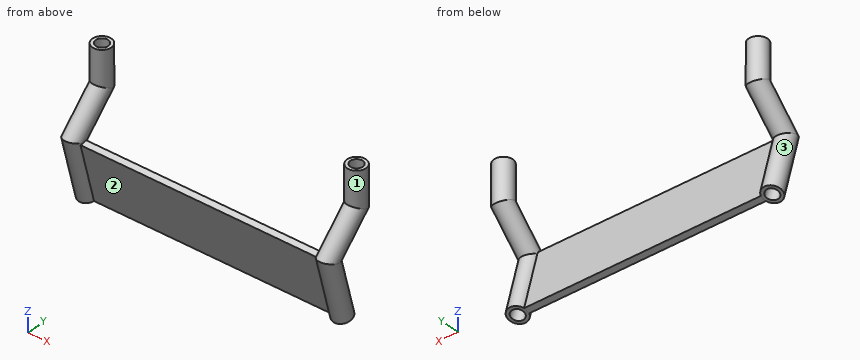
```python
from build123d import *

# Parameters (mm, degrees)
SWEEP_THIN1_PROFILE_R   = 30
SWEEP_THIN1_PROFILE_R_2 = 20
EXTRUDE_THIN1_START     = 20
EXTRUDE_THIN1_DEPTH     = 760


with BuildPart() as part:
    # Sweep-Thin1: sweep along a path in Sketch21
    with BuildLine(Plane(origin=(0, 0, 0), x_dir=(0, 0, -1), z_dir=(1, 0, 0))) as sweep_thin1_path:
        Line((0, 0), (120, 0))
        Line((120, 0), (226.066017178, -106.066017178))
        Line((226.066017178, -106.066017178), (419.251182436, -54.302208157))
    # Sweep-Thin1 profile (on start of the path) → Sweep-Thin1 (sweep)
    with BuildSketch(Plane(origin=(0, 0, 0), x_dir=(-1, 0, 0), z_dir=(0, 0, -1))):
        Circle(SWEEP_THIN1_PROFILE_R)
        Circle(SWEEP_THIN1_PROFILE_R_2, mode=Mode.SUBTRACT)
    sweep_thin1 = sweep(path=sweep_thin1_path.line, transition=Transition.RIGHT)

    # Sketch32 → Extrude-Thin1 (add)
    with BuildSketch(Plane(origin=(0, 0, 0), x_dir=(0, 0, -1), z_dir=(1, 0, 0)).offset(EXTRUDE_THIN1_START)):
        Polygon((228.654207629, -115.725275441), (421.839372887, -63.96146642), (416.662991985, -44.642949895), (223.477826727, -96.406758915), align=None)
    extrude(amount=EXTRUDE_THIN1_DEPTH)

    # Mirror1: Sweep-Thin1 across plane
    add(sweep_thin1.mirror(Plane(origin=(404.142135624, 0, 0), x_dir=(0, 0, 1), z_dir=(1, 0, 0))))


solid = part.part
```
Verification items for the finished model (mm, model axes). Face numbers are marked on the shaded views. A direction names the side the tool comes from. Give positions to 0.01 mm unless a question says otherwise; leave off trailing zeros. Loops run counter-clockwise (first coordinate to the right, second up) from the corner with the lowest first, then second, coordinate; pieces in that order, holes last.
1. Thickness scan on line 1 (Y direction, x = 0, z = -95); line 2 (X direction, y = 18.5, z = -112.5); line 3 (X direction, y = -60, z = -185.5). Record the ranges inside material, lowest first.
2. Section check A-A, the plane x = 0. Enter the section's corners in (y, z).
3. Section check B-B, the plane x = 700.5. Enter the section's corners in (y, z), then the cut area to 3 significant figures.
4. Section check C-C, the plane z = -364. Count the separate pieces of the cut face and the enclosed holes in it, then the cut area to 3 significant figures.
5. Set-up check for the marked faces 1, 2 and 3: record each of +Z, -Z, +X, -X, +Y, -Y from which the full face is reachable in a straight line by a thin tool's end or side.
6. Go/stop test with flat-tipped pins: pin 1 Ø3 at (x, y) = (331, -117.5) entering from +Z; pin 2 Ø1 at (x, z) = (345.5, -322.5) entering from +Y. Record where each tip stops, or that it passes through.
Geometry says:
1. line 1: y = -30 to -20, 20 to 30
1. line 2: x = -23.62 to -7.6, 7.6 to 23.62, 784.67 to 800.68, 815.88 to 831.9
1. line 3: x = -29.75 to -19.62, 19.62 to 29.75, 778.54 to 788.67, 827.9 to 838.03
2. outline: (-139.53, -217.1) - (-83.28, -427.02) - (-73.62, -424.43) - (-128.37, -220.09) - (-20, -111.72) - (-20, 0) - (-30, 0) - (-30, -107.57) - close; (-83.76, -232.04) - (-34.98, -414.07) - (-25.32, -411.49) - (-72.61, -235.03) - (30, -132.43) - (30, 0) - (20, 0) - (20, -128.28) - close
3. outline: (-115.73, -228.65) - (-63.96, -421.84) - (-44.64, -416.66) - (-96.41, -223.48) - close
3. area: 4,000 mm2
4. separate pieces: 1
4. enclosed holes: 2
4. area: 18,800 mm2
5. face 1: +Z
5. face 2: -Z, -Y
5. face 3: none
6. pin 1: passes through
6. pin 2: stops at y = -69.74
